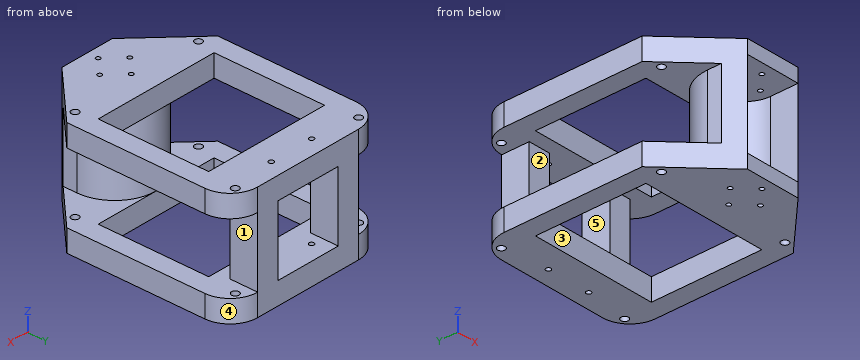
from build123d import *

# Parameters (mm, degrees)
SKETCH1_R           = 0.883567379
SKETCH1_R_2         = 0.896609669
SKETCH1_R_3         = 0.8
SKETCH1_R_4         = 1.35
BOSS_EXTRUDE1_DEPTH = 8
SKETCH2_W           = 8
SKETCH2_H           = 10
BOSS_EXTRUDE3_DEPTH = 25
BOSS_EXTRUDE4_START = 33
SKETCH1_2_R         = 0.883567379
SKETCH1_2_R_2       = 0.896609669
SKETCH1_2_R_3       = 0.8
SKETCH1_2_R_4       = 1.35
BOSS_EXTRUDE4_DEPTH = 8
CUT_EXTRUDE1_DEPTH  = 3
CUT_EXTRUDE2_START  = 28
CUT_EXTRUDE2_DEPTH  = 3
BOSS_EXTRUDE5_DEPTH = 25
CUT_EXTRUDE3_DEPTH  = 41
FILLET5_R           = 10
SKETCH8_W           = 46
SKETCH8_H           = 40
CUT_EXTRUDE4_DEPTH  = 79.4619407


with BuildPart() as part:
    # Sketch1 → Boss-Extrude1 (new body)
    with BuildSketch(Plane.XY):
        Polygon((-30, 20.206387144), (0, 20.206387144), (30, 20.206387144), (30, -59.793612856), (-30, -59.793612856), align=None)
        with Locations((-8, 14.206387144)):
            Circle(SKETCH1_R, mode=Mode.SUBTRACT)
        with Locations((8, 14.206387144)):
            Circle(SKETCH1_R_2, mode=Mode.SUBTRACT)
        with Locations((0, -43.793612856)):
            Circle(SKETCH1_R_3, mode=Mode.SUBTRACT)
        with Locations((6, -49.793612856)):
            Circle(SKETCH1_R_3, mode=Mode.SUBTRACT)
        with Locations((0, -55.793612856)):
            Circle(SKETCH1_R_3, mode=Mode.SUBTRACT)
        with Locations((-6, -49.793612856)):
            Circle(SKETCH1_R_3, mode=Mode.SUBTRACT)
        with Locations((-24.5, 16.206387144)):
            Circle(SKETCH1_R_4, mode=Mode.SUBTRACT)
        with Locations((24.5, 16.206387144)):
            Circle(SKETCH1_R_4, mode=Mode.SUBTRACT)
        with Locations((-24.5, -41.793612856)):
            Circle(SKETCH1_R_4, mode=Mode.SUBTRACT)
        with Locations((24.5, -41.793612856)):
            Circle(SKETCH1_R_4, mode=Mode.SUBTRACT)
    extrude(amount=BOSS_EXTRUDE1_DEPTH)

    # Sketch2 → Boss-Extrude3 (add)
    with BuildSketch(Plane.XY.offset(8)):
        with Locations((-16, 15.206387144)):
            Rectangle(SKETCH2_W, SKETCH2_H)
        with Locations((16, 15.206387144)):
            Rectangle(SKETCH2_W, SKETCH2_H)
    extrude(amount=BOSS_EXTRUDE3_DEPTH)

    # Sketch1<2> → Boss-Extrude4 (add)
    with BuildSketch(Plane.XY.offset(BOSS_EXTRUDE4_START)):
        Polygon((-30, 20.206387144), (0, 20.206387144), (30, 20.206387144), (30, -59.793612856), (-30, -59.793612856), align=None)
        with Locations((-8, 14.206387144)):
            Circle(SKETCH1_2_R, mode=Mode.SUBTRACT)
        with Locations((8, 14.206387144)):
            Circle(SKETCH1_2_R_2, mode=Mode.SUBTRACT)
        with Locations((0, -43.793612856)):
            Circle(SKETCH1_2_R_3, mode=Mode.SUBTRACT)
        with Locations((6, -49.793612856)):
            Circle(SKETCH1_2_R_3, mode=Mode.SUBTRACT)
        with Locations((0, -55.793612856)):
            Circle(SKETCH1_2_R_3, mode=Mode.SUBTRACT)
        with Locations((-6, -49.793612856)):
            Circle(SKETCH1_2_R_3, mode=Mode.SUBTRACT)
        with Locations((-24.5, 16.206387144)):
            Circle(SKETCH1_2_R_4, mode=Mode.SUBTRACT)
        with Locations((24.5, 16.206387144)):
            Circle(SKETCH1_2_R_4, mode=Mode.SUBTRACT)
        with Locations((-24.5, -41.793612856)):
            Circle(SKETCH1_2_R_4, mode=Mode.SUBTRACT)
        with Locations((24.5, -41.793612856)):
            Circle(SKETCH1_2_R_4, mode=Mode.SUBTRACT)
    extrude(amount=BOSS_EXTRUDE4_DEPTH)

    # Sketch3 → Cut-Extrude1 (cut)
    with BuildSketch(Plane.XY.offset(8)):
        with BuildLine():
            Line((-10, -49.793612856), (-10, -59.793612856))
            Line((-10, -59.793612856), (10, -59.793612856))
            Line((10, -59.793612856), (10, -49.793612856))
            ThreePointArc((10, -49.793612856), (0, -39.793612856), (-10, -49.793612856))
        make_face()
    extrude(amount=-CUT_EXTRUDE1_DEPTH, mode=Mode.SUBTRACT)

    # Sketch3<2> → Cut-Extrude2 (cut)
    with BuildSketch(Plane.XY.offset(8).offset(CUT_EXTRUDE2_START)):
        with BuildLine():
            Line((-10, -49.793612856), (-10, -59.793612856))
            Line((-10, -59.793612856), (10, -59.793612856))
            Line((10, -59.793612856), (10, -49.793612856))
            ThreePointArc((10, -49.793612856), (0, -39.793612856), (-10, -49.793612856))
        make_face()
    extrude(amount=-CUT_EXTRUDE2_DEPTH, mode=Mode.SUBTRACT)

    # Sketch5 → Boss-Extrude5 (add)
    with BuildSketch(Plane(origin=(0, 0, 33), x_dir=(-1, 0, 0), z_dir=(0, 0, -1))):
        with BuildLine():
            Line((-15, -49.793612856), (-15, -59.793612856))
            Line((-15, -59.793612856), (-10, -59.793612856))
            Line((-10, -59.793612856), (-10, -49.793612856))
            ThreePointArc((-10, -49.793612856), (0, -39.793612856), (10, -49.793612856))
            Line((10, -49.793612856), (10, -59.793612856))
            Line((10, -59.793612856), (15, -59.793612856))
            Line((15, -59.793612856), (15, -49.793612856))
            ThreePointArc((15, -49.793612856), (0, -34.793612856), (-15, -49.793612856))
        make_face()
    extrude(amount=BOSS_EXTRUDE5_DEPTH)

    # Sketch7 → Cut-Extrude3 (cut)
    with BuildSketch(Plane.XY.offset(41)):
        Polygon((30, -39.793612856), (30, -59.793612856), (10, -59.793612856), align=None)
        Polygon((-30, -39.793612856), (-30, -59.793612856), (-10, -59.793612856), align=None)
    extrude(amount=-CUT_EXTRUDE3_DEPTH, mode=Mode.SUBTRACT)

    # Fillet5
    fillet5_edges = [part.edges().sort_by_distance(p)[0] for p in [
        (-30, 20.206387144, 37),
        (-30, 20.206387144, 4),
        (30, 20.206387144, 4),
        (30, 20.206387144, 37),
    ]]
    fillet(fillet5_edges, radius=FILLET5_R)

    # Sketch8 → Cut-Extrude4 (cut, through all)
    with BuildSketch(Plane.XY.offset(41)):
        with Locations((0, -14.793612856)):
            Rectangle(SKETCH8_W, SKETCH8_H)
    extrude(amount=-CUT_EXTRUDE4_DEPTH, mode=Mode.SUBTRACT)


solid = part.part
Part model, mm, in its own coordinate system. Face numbers are marked on the shaded views. A direction names the side the tool comes from. Coordinates: 2 decimals unless noted, no trailing zeros. Write each loop counter-clockwise with the first axis right and the second up, starting at its lowest first coordinate (ties: lowest second). Pieces come first, ordered by that corner, then holes. Notation, with made-up numbers: M 76,17.25 L 117,17.25 A23 cw 117,51.25 Z; hole C -28.5,-27 d5. An arc over 180 degrees is marked long. Return JSON: item names as keys, results as strings.
1. Saw through at D-D, the plane z = 38.5. Count the separate pieces of the cut face and the enclosed holes in it, then the cut area to 3 significant figures.
Determined:
{"separate pieces": "1", "enclosed holes": "11", "area": "2,480 mm²"}
2. Saw through at C-C, the plane x = 8. Write the cut outline in (y, z), then the cut area to 3 significant figures.
Determined:
{"outline": "M -59.79,0 L -34.79,0 L -34.79,8 L -37.11,8 L -37.11,33 L -34.79,33 L -34.79,41 L -59.79,41 L -59.79,36 L -43.79,36 L -43.79,5 L -59.79,5 Z; M 5.21,0 L 13.31,0 L 13.31,8 L 5.21,8 Z; M 5.21,33 L 13.31,33 L 13.31,41 L 5.21,41 Z; M 15.1,0 L 20.21,0 L 20.21,8 L 15.1,8 Z; M 15.1,33 L 20.21,33 L 20.21,41 L 15.1,41 Z", "area": "683 mm²"}
3. Flat gauge pins, fed straight in: pin 1 Ø6 at (x, z) = (-15.5, 11.5) entering from -Y; pin 2 Ø4.5 at (x, y) = (-24.5, -41.79) entering from -Z; pin 3 Ø8 at (y, z) = (-55, 25) entering from +X; pin 4 Ø8 at (y, z) = (-54, 28) entering from -X. Where does each tip first touch, or does it go through?
Determined:
{"pin 1": "y = -57.29", "pin 2": "z = 0", "pin 3": "x = 15", "pin 4": "x = -15"}
4. Saw through at B-B, the plane x = 24.5. Write the cut outline in (y, z).
Determined:
{"outline": "M -45.29,0 L -43.14,0 L -43.14,8 L -45.29,8 Z; M -45.29,33 L -43.14,33 L -43.14,41 L -45.29,41 Z; M -40.44,0 L 14.86,0 L 14.86,8 L -40.44,8 Z; M -40.44,33 L 14.86,33 L 14.86,41 L -40.44,41 Z; M 17.56,0 L 19.14,0 L 19.14,8 L 17.56,8 Z; M 17.56,33 L 19.14,33 L 19.14,41 L 17.56,41 Z"}
5. Probe L1, parallel to Y at x = 6, z = 38.15; L2, parallel to Y at x = 8, z = 4.5; L3, parallel to X at y = 13, z = 25. List the from-to ranges inside material, lowest first.
Determined:
{"L1": "-59.79 to -50.59, -48.99 to -34.79, 5.21 to 20.21", "L2": "-59.79 to -34.79, 5.21 to 13.31, 15.1 to 20.21", "L3": "-20 to -12, 12 to 20"}
6. Saw through at A-A, the plane y = 0.5. Write the cut outline in (x, z), then the cut area to 3 significant figures.
Determined:
{"outline": "M -30,0 L -23,0 L -23,8 L -30,8 Z; M -30,33 L -23,33 L -23,41 L -30,41 Z; M 23,0 L 30,0 L 30,8 L 23,8 Z; M 23,33 L 30,33 L 30,41 L 23,41 Z", "area": "224 mm²"}
7. Pull direction Z, two halves, no side cores. Call the marked faces 4 and 5: pulls with the +Z half, pulls with the -Z half, needs draft (parallel to the pull), parting line crosses it, or undercut.
Determined:
{"face 4": "needs draft", "face 5": "undercut"}
8. 3-axis set-ups, long thin cutter, end or side, ignore diameter. For the marked faces 1, 2 and 3: which of +Z, -Z, +X, -X, +Y, -Y reach the whole face in a straight line?
Determined:
{"face 1": "+X, +Y, -Y", "face 2": "+X, -X", "face 3": "+Z, -Z"}
